The listing builds one solid part. Answer for the finished solid, in the listing's coordinates (mm). A direction names the side the tool comes from. Round coordinates to 2 decimals unless told otherwise and drop trailing zeros. Loops run counter-clockwise (first coordinate to the right, second up) from the corner with the lowest first, then second, coordinate; pieces in that order, holes last. Notation, with made-up numbers: (57.25, 78) -> (93.25, 78) arc R8 ccw to (93.25, 84) -> close; hole circle Ø2 at (60, 83). An arc over 180 degrees is marked (long way). Use a Markdown table: item, result. Add a question column.
Q1. Section D-D on x = 1.5 is taken. Give the vertices of the cut face in (y, z).
Q2. Consider line 1 (Z direction, x = -18.5, y = -10.5); line 2 (X direction, y = -21, z = 27.5); line 3 (Y direction, x = -31, z = 92). Determine where each line is inside the solid, lowest interval first.
Q3. Given pin 1 Ø3 at (x, z) = (30, 32) entering from +Y; pin 2 Ø8.5 at (y, z) = (-9.5, 35) entering from +X; pin 3 Ø8.5 at (y, z) = (-17.5, 32.5) entering from -X; pin 4 Ø1.5 at (x, y) = (8, 24.5) entering from +Z, each flat-ended and moving along its own axis, determine where each tip first touches the part or whether it passes through.
Q4. Section C-C on y = -20.5 is taken. Give the vertices of the cut face in (x, z), then the cut area to 3 significant figures.
Q5. Which of the six approach directions +Z, -Z, +X, -X, +Y, -Y give full straight-line access (tool end or side, diameter ignored) to faces 1 (the flat face through (-5, -18, 21)), 2 (the flat face through (1, 5, 10)), 3 (the flat face through (5, -18, 21))?
Q6. Section B-B on z = 15.5 is taken. Give the vertices of the cut face in (x, y).
Q7. Section A-A on x = 17 is taken. Give the vertices of the cut face in (y, z).
from build123d import *

# Parameters (mm, degrees)
BOSS_EXTRUDE1_DEPTH = 10
CHAMFER1_SIZE       = 10
SKETCH2_W           = 139.250997166
SKETCH2_H           = 9.771290108
BOSS_EXTRUDE2_DEPTH = 90
RIB1_REACH          = 129.722
SKETCH3_WALL_W      = 306.241984106
SKETCH3_WALL_H      = 10


with BuildPart() as part:
    # Sketch1 → Boss-Extrude1 (new body)
    with BuildSketch(Plane.XY):
        with BuildLine():
            Line((-42.118258456, 38.277525287), (69.625498583, 38.277525287))
            Line((69.625498583, 38.277525287), (69.625498583, -38.277525287))
            Line((69.625498583, -38.277525287), (-69.625498583, -38.277525287))
            Line((-69.625498583, -38.277525287), (-69.625498583, 10.77028516))
            ThreePointArc((-69.625498583, 10.77028516), (-61.568814481, 30.220841186), (-42.118258456, 38.277525287))
        make_face()
    extrude(amount=BOSS_EXTRUDE1_DEPTH)

    # Chamfer1
    chamfer1_edges = [part.edges().sort_by_distance(p)[0] for p in [
        (69.625498583, 38.277525287, 5),
    ]]
    chamfer(chamfer1_edges, length=CHAMFER1_SIZE)

    # Sketch2 → Boss-Extrude2 (add)
    with BuildSketch(Plane.XY.offset(10)):
        with Locations((0, -33.391880233)):
            Rectangle(SKETCH2_W, SKETCH2_H)
    extrude(amount=BOSS_EXTRUDE2_DEPTH)

    # Sketch3 wall → Rib1 (add, up to next)
    with BuildSketch(Plane(origin=(0, -14.25311759, 29.803162332), x_dir=(0, 0.584165456178, -0.811634597469), z_dir=(0, 0.811634597469, 0.584165456178)), mode=Mode.PRIVATE) as rib1_sk1:
        Rectangle(SKETCH3_WALL_W, SKETCH3_WALL_H)
    rib1_tool1 = extrude(rib1_sk1.sketch, amount=-RIB1_REACH, mode=Mode.PRIVATE) - part.part
    add(rib1_tool1.solids().sort_by_distance((0, -14.25311759, 29.803162332))[0])


solid = part.part
Checked values:
| question | item | result |
|---|---|---|
| 1 | outline | (-38.28, 0) -> (38.28, 0) -> (38.28, 10) -> (0, 10) -> (-28.51, 49.61) -> (-28.51, 100) -> (-38.28, 100) -> close |
| 2 | line 1 | z = 0 to 10 |
| 2 | line 2 | x = -5 to 5 |
| 2 | line 3 | y = -38.28 to -28.51 |
| 3 | pin 1 | stops at y = -28.51 |
| 3 | pin 2 | passes through |
| 3 | pin 3 | stops at x = -5 |
| 3 | pin 4 | stops at z = 10 |
| 4 | outline | (-69.63, 0) -> (69.63, 0) -> (69.63, 10) -> (5, 10) -> (5, 38.48) -> (-5, 38.48) -> (-5, 10) -> (-69.63, 10) -> close |
| 4 | area | 1,680 mm2 |
| 5 | face 1 | +Z, -X, +Y |
| 5 | face 2 | +Z, +Y |
| 5 | face 3 | +Z, +X, +Y |
| 6 | outline | (-69.63, -38.28) -> (69.63, -38.28) -> (69.63, -28.51) -> (5, -28.51) -> (5, -3.96) -> (-5, -3.96) -> (-5, -28.51) -> (-69.63, -28.51) -> close |
| 7 | outline | (-38.28, 0) -> (38.28, 0) -> (38.28, 10) -> (-28.51, 10) -> (-28.51, 100) -> (-38.28, 100) -> close |
